Geometry check sheet. Reference: drawing and pictorial views, mm from the part's lowest x, y, z. A direction names the side the tool comes from. Give positions to 0.01 mm unless a question says otherwise; leave off trailing zeros. Write each loop counter-clockwise with the first axis right and the second up, starting at its lowest first coordinate (ties: lowest second). Pieces come first, ordered by that corner, then holes. Notation, with made-up numbers: (6, 77) -> (45, 77) arc R15 ccw to (45, 104) -> close; hole circle Ø11 at (34, 44.5). An arc over 180 degrees is marked (long way). Use a Markdown table: item, result. Add a question column.
1. Cross-section at D-D (z = 5). Enter the section's corners in (x, y), then the cut area to 3 significant figures.
2. Cross-section at A-A (x = 50). Enter the section's corners in (y, z).
3. Set-up check for the marked faces 1, 2 and 3: record each of +Z, -Z, +X, -X, +Y, -Y from which the full face is reachable in a straight line by a thin tool's end or side.
4. Cross-section at C-C (x = 92). Enter the section's corners in (y, z).
5. Cross-section at B-B (y = 44.5). Enter the section's corners in (x, z).
6. Release check for a two-part mould opening along Z. For the marked faces 4, 5 and 6 record: released by +Z, released by -Z, zero draft, split by the parting line, or undercut.
7. Gauge pin test, flat ends, axial feed: P1, Ø1, axis at x = 23, y = 42.5, coming from the -Z side; P2, Ø18, axis at x = 50, y = 40, coming from the +Z side. Record the tip position at first contact, or that the pin passes through.
8. Scan lines: probe 1 along Z at (x, y) = (75, 36); probe 2 along X at (y, z) = (40, 10.5); probe 3 along Y at (x, z) = (50, 48). Record each from-to range of solid material in increasing order. Write a range as [from, to].
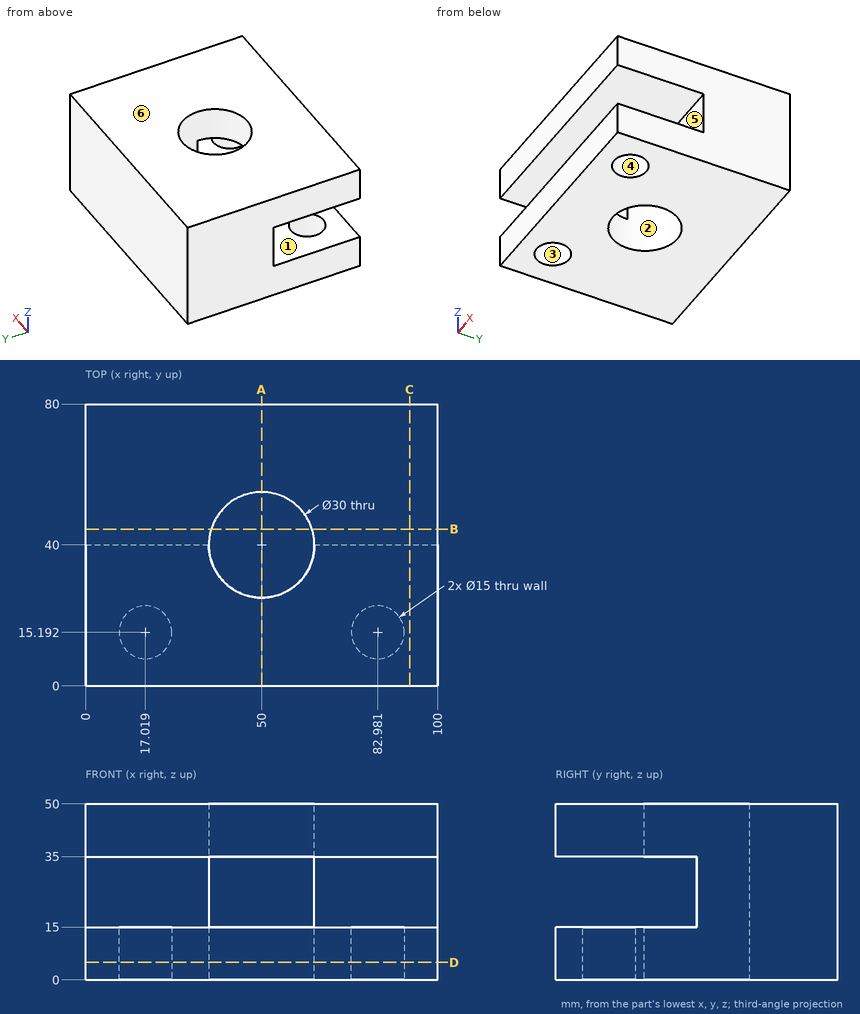
Worked answers:
| question | item | result |
|---|---|---|
| 1 | outline | (0, 0) -> (100, 0) -> (100, 80) -> (0, 80) -> close; hole circle Ø15 at (17.02, 15.19); hole circle Ø30 at (50, 40); hole circle Ø15 at (82.98, 15.19) |
| 1 | area | 6,940 mm² |
| 2 | outline | (0, 0) -> (25, 0) -> (25, 15) -> (0, 15) -> close; (0, 35) -> (25, 35) -> (25, 50) -> (0, 50) -> close; (55, 0) -> (80, 0) -> (80, 50) -> (55, 50) -> close |
| 3 | face 1 | +X, -X, -Y |
| 3 | face 2 | +Z, -Z |
| 3 | face 3 | -Z |
| 4 | outline | (0, 0) -> (80, 0) -> (80, 50) -> (0, 50) -> (0, 35) -> (40, 35) -> (40, 15) -> (0, 15) -> close |
| 5 | outline | (0, 0) -> (35.69, 0) -> (35.69, 50) -> (0, 50) -> close; (64.31, 0) -> (100, 0) -> (100, 50) -> (64.31, 50) -> close |
| 6 | face 4 | zero draft |
| 6 | face 5 | undercut |
| 6 | face 6 | released by +Z |
| 7 | P1 | stops at z = 0 |
| 7 | P2 | passes through |
| 8 | probe 1 | z = [0, 15], [35, 50] |
| 8 | probe 2 | x = [0, 35], [65, 100] |
| 8 | probe 3 | y = [0, 25], [55, 80] |
